```python
from build123d import *

# Parameters (mm, degrees)
PAD051_DEPTH    = 57
POCKET043_DEPTH = 16
POCKET042_DEPTH = 16
SKETCH097_R     = 13
POCKET047_DEPTH = 10.001
PAD052_DEPTH    = 25


with BuildPart() as part:
    # Sketch095 → Pad051 (new body)
    with BuildSketch(Plane.YZ):
        Polygon((92.056432, 72.85), (207.943568, 72.85), (213.208897, 62.85), (86.791103, 62.85), align=None)
    extrude(amount=-PAD051_DEPTH)

    # Sketch098 (on Face5 of Pad051) → Pocket043 (cut)
    with BuildSketch(Plane.YZ):
        Polygon((86.791103, 62.85), (98.092594, 62.85), (103.357923, 72.85), (92.056432, 72.85), align=None)
        Polygon((207.943568, 72.85), (196.642077, 72.85), (201.907406, 62.85), (213.208897, 62.85), align=None)
    extrude(amount=-POCKET043_DEPTH, mode=Mode.SUBTRACT)

    # Sketch096 (on Face8 of Pocket043) → Pocket042 (cut)
    with BuildSketch(Plane(origin=(-57, 0, 0), x_dir=(0, 1, 0), z_dir=(-1, 0, 0))):
        Polygon((86.791103, -62.85), (92.056432, -72.85), (103.357923, -72.85), (98.092594, -62.85), align=None)
        Polygon((201.907406, -62.85), (213.208897, -62.85), (207.943568, -72.85), (196.642077, -72.85), align=None)
    extrude(amount=-POCKET042_DEPTH, mode=Mode.SUBTRACT)

    # Sketch097 (on Face1 of Pocket042) → Pocket047 (cut, through all)
    with BuildSketch(Plane(origin=(0, 0, 72.85), x_dir=(0, -1, 0), z_dir=(0, 0, 1))):
        with Locations((-150, -28.5)):
            Circle(SKETCH097_R)
    extrude(amount=-POCKET047_DEPTH, mode=Mode.SUBTRACT)

    # Sketch104 (on Face1 of Pocket047) → Pad052 (join)
    with BuildSketch(Plane(origin=(0, 0, 72.85), x_dir=(0, -1, 0), z_dir=(0, 0, 1))):
        Polygon((-176.25, -2.25), (-176.25, -17.25), (-171.25, -17.25), (-171.25, -7.25), (-161.25, -7.25), (-161.25, -2.25), align=None)
        Polygon((-128.75, -7.25), (-128.75, -17.25), (-123.75, -17.25), (-123.75, -2.25), (-138.75, -2.25), (-138.75, -7.25), align=None)
        Polygon((-138.75, -54.75), (-123.75, -54.75), (-123.75, -39.75), (-128.75, -39.75), (-128.75, -49.75), (-138.75, -49.75), align=None)
        Polygon((-171.25, -49.75), (-161.25, -49.75), (-161.25, -54.75), (-176.25, -54.75), (-176.25, -39.75), (-171.25, -39.75), align=None)
    extrude(amount=PAD052_DEPTH)


solid = part.part
```
Geometry: final body of the model. Coordinates: model frame, mm. A direction names the side the tool comes from. Coordinates: 2 decimals unless noted, no trailing zeros. Order: outer loops, then holes, each group sorted by start corner. A loop starts at its lowest first (then second) coordinate and runs counter-clockwise, first axis right, second up.
Item 1: Draft query along X for faces 6 (the face through (-2.25, 169, 85)), 7 (the face through (-10, 123.75, 85)), 8 (the face through (-17.25, 174, 85)). Return one class per face: released by +X, released by -X, zero draft, split by the parting line, or undercut.
Answer:
face 6: released by +X
face 7: zero draft
face 8: undercut
Item 2: Section query A-A (y = 150). Output: boundary loops of the cut face in (x, z).
Answer:
outline: (-57, 62.85) - (-41.5, 62.85) - (-41.5, 72.85) - (-57, 72.85) - close; (-15.5, 62.85) - (0, 62.85) - (0, 72.85) - (-15.5, 72.85) - close
Item 3: Section query B-B (x = -28.5). Output: boundary loops of the cut face in (y, z).
Answer:
outline: (86.79, 62.85) - (137, 62.85) - (137, 72.85) - (92.06, 72.85) - close; (163, 62.85) - (213.21, 62.85) - (207.94, 72.85) - (163, 72.85) - close
Item 4: Contact query for flat-ended pins moving along their axis: P1, Ø8, axis at y = 93.5, z = 69.5, coming from the -X side; P2, Ø4.5, axis at y = 168, z = 82.5, coming from the +X side; P3, Ø2.5, axis at x = -6, z = 89, coming from the +Y side. Output: stop coordinate, or through.
Answer:
P1: stops at x = -41
P2: stops at x = -2.25
P3: stops at y = 176.25
Item 5: Material intervals for line 1 along X through (y, z) = (138, 89); line 2 along X through (y, z) = (175.5, 92.5); line 3 along Z through (x, y) = (-47.5, 158), sorted ascending.
Answer:
line 1: x = -54.75 to -49.75, -7.25 to -2.25
line 2: x = -54.75 to -39.75, -17.25 to -2.25
line 3: z = 62.85 to 72.85
Item 6: Section query D-D (z = 66). Output: boundary loops of the cut face in (x, y), then the cut area to 3 significant figures.
Answer:
outline: (-57, 99.75) - (-41, 99.75) - (-41, 88.45) - (-16, 88.45) - (-16, 99.75) - (0, 99.75) - (0, 200.25) - (-16, 200.25) - (-16, 211.55) - (-41, 211.55) - (-41, 200.25) - (-57, 200.25) - close; hole circle Ø26 at (-28.5, 150)
area: 5,760 mm2
Item 7: Section query C-C (z = 75). Output: boundary loops of the cut face in (x, y), then the cut area to 3 significant figures.
Answer:
outline: (-54.75, 123.75) - (-39.75, 123.75) - (-39.75, 128.75) - (-49.75, 128.75) - (-49.75, 138.75) - (-54.75, 138.75) - close; (-54.75, 161.25) - (-49.75, 161.25) - (-49.75, 171.25) - (-39.75, 171.25) - (-39.75, 176.25) - (-54.75, 176.25) - close; (-17.25, 123.75) - (-2.25, 123.75) - (-2.25, 138.75) - (-7.25, 138.75) - (-7.25, 128.75) - (-17.25, 128.75) - close; (-17.25, 171.25) - (-7.25, 171.25) - (-7.25, 161.25) - (-2.25, 161.25) - (-2.25, 176.25) - (-17.25, 176.25) - close
area: 500 mm2
Item 8: Access query for faces 1 (the face through (-41, 95, 68)), 2 (the face through (-52, 138.75, 85)), 3 (the face through (-39.75, 126, 85)), 4 (the face through (-7.9, 100.7, 67.8)), 5 (the face through (-12, 171.25, 85)). Directions: +Z, -Z, +X, -X, +Y, -Y. A direction counts if a zero-diameter tool reaches every point of the face in a straight line with its end or side. Return the directions, or none.
Answer:
face 1: +Z, -X, -Y
face 2: +Z, +X, -X
face 3: +Z, +Y, -Y
face 4: +Z, +X, -Y
face 5: +Z
